from build123d import *

# Parameters (mm, degrees)
SKETCH1_R           = 2
SKETCH1_R_2         = 1
BOSS_EXTRUDE1_DEPTH = 4
SKETCH2_R           = 1.1
CUT_EXTRUDE1_DEPTH  = 2
SKETCH3_W           = 14.966629548
SKETCH3_H           = 2
CUT_EXTRUDE2_DEPTH  = 23
FILLET1_R           = 3
FILLET2_R           = 2
FILLET3_R           = 2
SKETCH4_R           = 2.5
SKETCH4_R_2         = 1.1
BOSS_EXTRUDE2_DEPTH = 2


with BuildPart() as part:
    # Sketch1 → Boss-Extrude1 (new body)
    # profile 1 of 9: a face of its own
    with BuildSketch(Plane(origin=(0, 0, 0), x_dir=(1, 0, 0), z_dir=(0, 1, 0))):
        with BuildLine():
            Line((-14, 3), (-8.485281374, 3))
            ThreePointArc((-8.485281374, 3), (-8.04667731, 4.031250956), (-7.483314774, 5))
            Line((-7.483314774, 5), (-14, 5))
            Line((-14, 5), (-14, 3))
        make_face()
    # profile 2 of 9: a face of its own
    with BuildSketch(Plane(origin=(0, 0, 0), x_dir=(1, 0, 0), z_dir=(0, 1, 0))):
        with BuildLine():
            ThreePointArc((-7.483314774, 5), (-8.04667731, 4.031250956), (-8.485281374, 3))
            Line((-8.485281374, 3), (-6.32455532, 3))
            ThreePointArc((-6.32455532, 3), (-5.700169593, 4.063012013), (-4.898979486, 5))
            Line((-4.898979486, 5), (-7.483314774, 5))
        make_face()
    # profile 3 of 9: a face of its own
    with BuildSketch(Plane(origin=(0, 0, 0), x_dir=(1, 0, 0), z_dir=(0, 1, 0))):
        with BuildLine():
            ThreePointArc((4.898979486, 5), (5.700169593, 4.063012013), (6.32455532, 3))
            Line((6.32455532, 3), (8.485281374, 3))
            ThreePointArc((8.485281374, 3), (8.04667731, 4.031250956), (7.483314774, 5))
            Line((7.483314774, 5), (4.898979486, 5))
        make_face()
    # profile 4 of 9: a face of its own
    with BuildSketch(Plane(origin=(0, 0, 0), x_dir=(1, 0, 0), z_dir=(0, 1, 0))):
        with BuildLine():
            ThreePointArc((7.483314774, 5), (0, 9), (-7.483314774, 5))
            Line((-7.483314774, 5), (-4.898979486, 5))
            ThreePointArc((-4.898979486, 5), (0, 7), (4.898979486, 5))
            Line((4.898979486, 5), (7.483314774, 5))
        make_face()
    # profile 5 of 9: a face of its own
    with BuildSketch(Plane(origin=(0, 0, 0), x_dir=(1, 0, 0), z_dir=(0, 1, 0))):
        with BuildLine():
            Line((-1.803943959, 16.863589134), (-7.483314774, 5))
            ThreePointArc((-7.483314774, 5), (0, 9), (7.483314774, 5))
            Line((7.483314774, 5), (1.803943959, 16.863589134))
            ThreePointArc((1.803943959, 16.863589134), (1.950370211, 16.44278216), (2, 16))
            ThreePointArc((2, 16), (-0.44278216, 14.049629789), (-1.803943959, 16.863589134))
        make_face()
    # profile 6 of 9: a face of its own
    with BuildSketch(Plane(origin=(0, 0, 0), x_dir=(1, 0, 0), z_dir=(0, 1, 0))):
        with BuildLine():
            Line((14, 5), (7.483314774, 5))
            ThreePointArc((7.483314774, 5), (8.04667731, 4.031250956), (8.485281374, 3))
            Line((8.485281374, 3), (14, 3))
            Line((14, 3), (14, 5))
        make_face()
    # profile 7 of 9: a face of its own
    with BuildSketch(Plane(origin=(0, 0, 0), x_dir=(1, 0, 0), z_dir=(0, 1, 0))):
        with BuildLine():
            ThreePointArc((-7.483314774, 5), (-8.04667731, 4.031250956), (-8.485281374, 3))
            Line((-8.485281374, 3), (-6.32455532, 3))
            ThreePointArc((-6.32455532, 3), (-5.700169593, 4.063012013), (-4.898979486, 5))
            Line((-4.898979486, 5), (-7.483314774, 5))
        make_face()
    # profile 8 of 9: a face of its own
    with BuildSketch(Plane(origin=(0, 0, 0), x_dir=(1, 0, 0), z_dir=(0, 1, 0))):
        with BuildLine():
            ThreePointArc((4.898979486, 5), (5.700169593, 4.063012013), (6.32455532, 3))
            Line((6.32455532, 3), (8.485281374, 3))
            ThreePointArc((8.485281374, 3), (8.04667731, 4.031250956), (7.483314774, 5))
            Line((7.483314774, 5), (4.898979486, 5))
        make_face()
    # profile 9 of 9: a face of its own
    with BuildSketch(Plane(origin=(0, 0, 0), x_dir=(1, 0, 0), z_dir=(0, 1, 0))):
        with Locations((0, 16)):
            Circle(SKETCH1_R)
        with Locations(Location((0, 16, 0), (0, 0, 270))):
            Circle(SKETCH1_R_2, mode=Mode.SUBTRACT)
    extrude(amount=BOSS_EXTRUDE1_DEPTH)

    # Sketch2 → Cut-Extrude1 (cut)
    with BuildSketch(Plane(origin=(0, 0, -5), x_dir=(-1, 0, 0), z_dir=(0, 0, -1))):
        with Locations((-12, 2)):
            Circle(SKETCH2_R)
        with Locations((12, 2)):
            Circle(SKETCH2_R)
    extrude(amount=-CUT_EXTRUDE1_DEPTH, mode=Mode.SUBTRACT)

    # Sketch3 → Cut-Extrude2 (cut)
    with BuildSketch(Plane(origin=(0, 0, -5), x_dir=(-1, 0, 0), z_dir=(0, 0, -1))):
        with Locations((0, 3)):
            Rectangle(SKETCH3_W, SKETCH3_H)
    extrude(amount=CUT_EXTRUDE2_DEPTH, mode=Mode.SUBTRACT)

    # Fillet1
    fillet1_edges = [part.edges().sort_by_distance(p)[0] for p in [
        (-7.483314774, 1, -5),
        (7.483314774, 1, -5),
    ]]
    fillet(fillet1_edges, radius=FILLET1_R)

    # Fillet2
    fillet2_edges = [part.edges().sort_by_distance(p)[0] for p in [
        (-14, 0, -4),
        (14, 0, -4),
        (14, 4, -4),
        (-14, 4, -4),
    ]]
    fillet(fillet2_edges, radius=FILLET2_R - 0.0001)  # a hair under: the kernel refuses the full size

    # Fillet3
    fillet3_edges = [part.edges().sort_by_distance(p)[0] for p in [
        (7.13608574, 2, -5),
        (-7.13608574, 2, -5),
    ]]
    fillet(fillet3_edges, radius=FILLET3_R - 0.0001)  # a hair under: the kernel refuses the full size

    # Sketch4 → Boss-Extrude2 (add)
    # profile 1 of 2: a face of its own
    with BuildSketch(Plane(origin=(0, 0, -5), x_dir=(-1, 0, 0), z_dir=(0, 0, -1))):
        with Locations((12, 2)):
            Circle(SKETCH4_R)
        with Locations((12, 2)):
            Circle(SKETCH4_R_2, mode=Mode.SUBTRACT)
    # profile 2 of 2: a face of its own
    with BuildSketch(Plane(origin=(0, 0, -5), x_dir=(-1, 0, 0), z_dir=(0, 0, -1))):
        with Locations((-12, 2)):
            Circle(SKETCH4_R)
        with Locations((-12, 2)):
            Circle(SKETCH4_R_2, mode=Mode.SUBTRACT)
    extrude(amount=-BOSS_EXTRUDE2_DEPTH)


solid = part.part
Verification items for the finished model (mm, model axes). A direction names the side the tool comes from. Round coordinates to 2 decimals unless told otherwise and drop trailing zeros. Loops run counter-clockwise (first coordinate to the right, second up) from the corner with the lowest first, then second, coordinate; pieces in that order, holes last. Notation, with made-up numbers: M 63.25,-19 L 104.25,-19 A10 cw 104.25,-7 Z; hole C -28,45 d8. An arc over 180 degrees is marked long. Write each question's results on one line, items separated by ' | '.
1) Gauge pin test, flat ends, axial feed: P1, Ø2, axis at x = 3, z = -8, coming from the +Y side; P2, Ø1, axis at x = -6.5, z = -4.5, coming from the +Y side; P3, Ø2.5, axis at x = 12, y = 2, coming from the -Z side. Record the tip position at first contact, or that the pin passes through.
Checks:
P1: stops at y = 2 | P2: stops at y = 4 | P3: stops at z = -5
2) Section check A-A on x = 12. Record the boundary of the cut face in (y, z), then the cut area to 3 significant figures.
Checks:
outline: M -0.5,-5 L 0.9,-5 L 0.9,-3 L -0.5,-3 Z; M 3.1,-5 L 4.5,-5 L 4.5,-3 L 3.1,-3 Z | area: 5.60 mm2
3) Section check C-C on y = 1.35. Record the boundary of the cut face in (x, z), then the cut area to 3 significant figures.
Checks:
outline: M -14.41,-5 L -12.89,-5 L -12.89,-3 L -14.41,-3 Z; M -11.11,-5 L -9.37,-5 A3 cw -6.67,-6.7 L -1.8,-16.86 A2 ccw 1.8,-16.86 L 6.67,-6.7 A3 cw 9.37,-5 L 11.11,-5 L 11.11,-3 L 6.32,-3 A7 cw -6.32,-3 L -11.11,-3 Z; M 12.89,-5 L 14.41,-5 L 14.41,-3 L 12.89,-3 Z; hole C 0,-16 d2 | area: 125 mm2
4) Scan lines: L1, parallel to Y at x = 12, z = -4; L2, parallel to X at y = 1, z = -4.5; L3, parallel to Z at x = 0, y = 0.6. Record each from-to range of solid material in increasing order. Write a range as from..to.
Checks:
L1: y = -0.5..0.9, 3.1..4.5 | L2: x = -14.29..-12.46, -11.54..-5.36, 5.36..11.54, 12.46..14.29 | L3: z = -18..-17, -15..-7
5) Mould release check, pull along X, two halves, no side actions. Record for faces 1 (the flat face through (0, 0, -9)), 2 (the flat face through (0, 2, -11)), 3 (the flat face through (-4.2, 1, -11.86)), 4 (the cylindrical face through (10.984, 1.579, -4.014)): released by +X, released by -X, zero draft, split by the parting line, or undercut.
Checks:
face 1: undercut | face 2: zero draft | face 3: released by -X | face 4: undercut
6) Section check B-B on z = -3.75. Record the boundary of the cut face in (x, y).
Checks:
outline: M -10.5,0 L -5.91,0 L -5.91,4 L -10.5,4 A2.5 ccw long Z; M 5.91,0 L 10.5,0 A2.5 ccw long 10.5,4 L 5.91,4 Z; hole C -12,2 d2.2; hole C 12,2 d2.2
7) Access from +Z, -Z, +X, -X, +Y, -Y to the whole of each face (thin tool, end or side, straight path). Record for faces 5 (the flat face through (-10.7, 2, -5)), 6 (the flat face through (-8, 4, -4)), 7 (the flat face through (11, 3, -5)), 8 (the cylindrical face through (0, 1, -18)).
Checks:
face 5: -Z, -X, +Y, -Y | face 6: +Z, -Z, +Y | face 7: -Z, +X, +Y, -Y | face 8: -Z, +Y, -Y
8) Section check D-D on z = -16. Record the boundary of the cut face in (x, y), then the cut area to 3 significant figures.
Checks:
outline: M -2.22,0 L -1,0 L -1,2 L -2.22,2 Z; M 1,0 L 2.22,0 L 2.22,2 L 1,2 Z | area: 4.87 mm2
